from build123d import *

# Parameters (mm, degrees)
EXTRUDE_1_DEPTH = 12
M6X1_0_1_D      = 5
M6X1_0_1_DEPTH  = 15
M6X1_0_1_TIP    = 1.502151548


with BuildPart() as part:
    # 草圖1 → 填料-伸長1 (new body)
    with BuildSketch(Plane.XY):
        with BuildLine():
            Line((-5, 0), (5, 0))
            Line((5, 0), (5, -3))
            ThreePointArc((5, -3), (0, -4.339745962), (-5, -3))
            Line((-5, -3), (-5, 0))
        make_face()
    extrude(amount=EXTRUDE_1_DEPTH)

    # M6x1.0 螺紋孔1
    with Locations(Plane(origin=(0, 0, 0), x_dir=(1, 0, 0), z_dir=(0, 1, 0))):
        with Locations((0, -6)):
            Hole(M6X1_0_1_D / 2, depth=M6X1_0_1_DEPTH)
            with Locations((0, 0, -(M6X1_0_1_DEPTH + M6X1_0_1_TIP / 2))):  # 118° drill point
                Cone(0, M6X1_0_1_D / 2, M6X1_0_1_TIP, mode=Mode.SUBTRACT)


solid = part.part
Read the model definition and answer for the solid it produces. Units are mm, in the model's axes. Give positions to 0.01 mm unless a question says otherwise; leave off trailing zeros. Loops run counter-clockwise (first coordinate to the right, second up) from the corner with the lowest first, then second, coordinate; pieces in that order, holes last. Notation, with made-up numbers: M 10,-12 L 46,-12 A7 cw 46,0 Z; hole C 86.25,14.25 d11. An arc over 180 degrees is marked long. Write each question's results on one line, items separated by ' | '.
1. Section A-A on x = 0 is taken. Give the vertices of the cut face in (y, z).
Values:
outline: M -4.34,0 L 0,0 L 0,3.5 L -4.34,3.5 Z; M -4.34,8.5 L 0,8.5 L 0,12 L -4.34,12 Z
2. Given pin 1 (3 mm diameter, centred on x = -1.5, z = 6, fed in from -Y); pin 2 (1.5 mm diameter, centred on x = -1, z = 7, fed in from +Y); pin 3 (1 mm diameter, centred on x = -4, z = 6, fed in from -Y), each flat-ended and moving along its own axis, determine where each tip first touches the part or whether it passes through.
Values:
pin 1: stops at y = -4.12 | pin 2: passes through | pin 3: stops at y = -3.71
3. The mould has two halves that part along Z. Classify faces 1 (the face through (0, -2, 0)), 2 (the face through (2.5, -2.2, 5.9)), 3 (the face through (-5, -2, 6)), 4 (the face through (0, -2, 12)): pulls with the +Z half, pulls with the -Z half, needs draft (parallel to the pull), parting line crosses it, or undercut.
Values:
face 1: pulls with the -Z half | face 2: undercut | face 3: needs draft | face 4: pulls with the +Z half
4. Section C-C on y = -2.2 is taken. Give the vertices of the cut face in (x, z), plus the area to 3 significant figures.
Values:
outline: M -5,0 L 5,0 L 5,12 L -5,12 Z; hole C 0,6 d5 | area: 100 mm^2
5. Straight lines are drawn through the part: line 1 (Z direction, x = 0, y = -1); line 2 (X direction, y = -0.55, z = 3.75); line 3 (Z direction, x = -0.5, y = -2.5). For each, find the intervals that lie inside material, in ascending order. Write a range as [from, to].
Values:
line 1: z = [0, 3.5], [8.5, 12] | line 2: x = [-5, -1.09], [1.09, 5] | line 3: z = [0, 3.55], [8.45, 12]
6. Section D-D on z = 2 is taken. Give the vertices of the cut face in (x, y), plus the area to 3 significant figures.
Values:
outline: M -5,-3 A10 ccw 5,-3 L 5,0 L -5,0 Z | area: 39.1 mm^2
7. Section B-B on z = 6 is taken. Give the vertices of the cut face in (x, y), plus the area to 3 significant figures.
Values:
outline: M -5,-3 A10 ccw -2.5,-4.02 L -2.5,0 L -5,0 Z; M 2.5,-4.02 A10 ccw 5,-3 L 5,0 L 2.5,0 Z | area: 17.9 mm^2
